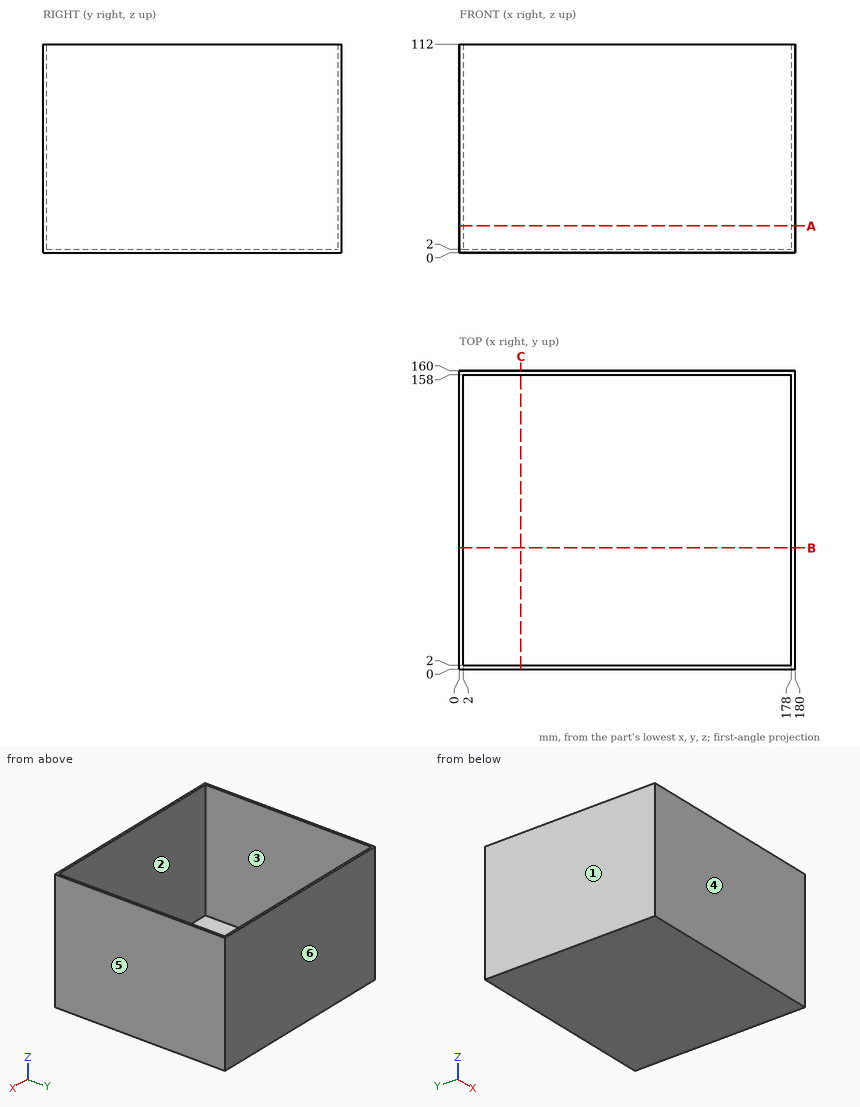
Verification items for this drawing (mm, ordinates from the low corner). A direction names the side the tool comes from. Give positions to 0.01 mm unless a question says otherwise; leave off trailing zeros. Write each loop counter-clockwise with the first axis right and the second up, starting at its lowest first coordinate (ties: lowest second). Pieces come first, ordered by that corner, then holes.
1) Set-up check for the marked faces 1 and 2: record each of +Z, -Z, +X, -X, +Y, -Y from which the full face is reachable in a straight line by a thin tool's end or side.
Values follow:
face 1: +Z, -Z, -X, +Y, -Y
face 2: +Z
2) Release check for a two-part mould opening along Y. For the marked faces 3, 4, 5 and 6 record: released by +Y, released by -Y, zero draft, split by the parting line, or undercut.
Values follow:
face 3: undercut
face 4: released by -Y
face 5: zero draft
face 6: released by +Y
3) Thickness scan on line 1 (X direction, y = 53.5, z = 32); line 2 (Y direction, x = 125.5, z = 43.5); line 3 (Z direction, x = 62, y = 81). Record the ranges inside material, lowest first.
Values follow:
line 1: x = 0 to 2, 178 to 180
line 2: y = 0 to 2, 158 to 160
line 3: z = 0 to 2
4) Cross-section at C-C (x = 33). Record the boundary of the cut face in (y, z).
Values follow:
outline: (0, 0) - (160, 0) - (160, 112) - (158, 112) - (158, 2) - (2, 2) - (2, 112) - (0, 112) - close
5) Cross-section at B-B (y = 65). Record the boundary of the cut face in (x, z), plus the area to 3 significant figures.
Values follow:
outline: (0, 0) - (180, 0) - (180, 112) - (178, 112) - (178, 2) - (2, 2) - (2, 112) - (0, 112) - close
area: 800 mm2
6) Go/stop test with a flat-tipped pin: pin 1 Ø3 at (x, y) = (150, 114.5) entering from +Z. Record where the tip stops, or that it passes through.
Values follow:
pin 1: stops at z = 2
7) Cross-section at A-A (z = 14.5). Record the boundary of the cut face in (x, y).
Values follow:
outline: (0, 0) - (180, 0) - (180, 160) - (0, 160) - close; hole (2, 2) - (178, 2) - (178, 158) - (2, 158) - close
